```python
from build123d import *

# Parameters (mm, degrees)
SKETCH1_W           = 35.5
SKETCH1_H           = 37
SKETCH1_W_2         = 31.32
SKETCH1_H_2         = 15.62
BOSS_EXTRUDE1_DEPTH = 3
SKETCH2_W           = 35.5
SKETCH2_H           = 10
SKETCH2_R           = 1.65
BOSS_EXTRUDE2_DEPTH = 3


with BuildPart() as part:
    # Sketch1 → Boss-Extrude1 (new body)
    with BuildSketch(Plane.XY):
        with Locations((17.75, 18.5)):
            Rectangle(SKETCH1_W, SKETCH1_H)
        with BuildLine():
            Line((4.5, 35.95), (5.6, 35.95))
            ThreePointArc((5.6, 35.95), (6.7, 34.85), (5.6, 33.75))
            Line((5.6, 33.75), (4.5, 33.75))
            ThreePointArc((4.5, 33.75), (3.4, 34.85), (4.5, 35.95))
        make_face(mode=Mode.SUBTRACT)
        with BuildLine():
            Line((29.9, 35.95), (31, 35.95))
            ThreePointArc((31, 35.95), (32.1, 34.85), (31, 33.75))
            Line((31, 33.75), (29.9, 33.75))
            ThreePointArc((29.9, 33.75), (28.8, 34.85), (29.9, 35.95))
        make_face(mode=Mode.SUBTRACT)
        with BuildLine():
            Line((29.9, 8.25), (31, 8.25))
            ThreePointArc((31, 8.25), (32.1, 7.15), (31, 6.05))
            Line((31, 6.05), (29.9, 6.05))
            ThreePointArc((29.9, 6.05), (28.8, 7.15), (29.9, 8.25))
        make_face(mode=Mode.SUBTRACT)
        with BuildLine():
            Line((4.5, 8.25), (5.6, 8.25))
            ThreePointArc((5.6, 8.25), (6.7, 7.15), (5.6, 6.05))
            Line((5.6, 6.05), (4.5, 6.05))
            ThreePointArc((4.5, 6.05), (3.4, 7.15), (4.5, 8.25))
        make_face(mode=Mode.SUBTRACT)
        with Locations((17.75, 23.05)):
            Rectangle(SKETCH1_W_2, SKETCH1_H_2, mode=Mode.SUBTRACT)
    extrude(amount=BOSS_EXTRUDE1_DEPTH)

    # Sketch2 → Boss-Extrude2 (add)
    with BuildSketch(Plane.XZ):
        with Locations((17.75, 8)):
            Rectangle(SKETCH2_W, SKETCH2_H)
        with Locations(Location((3.75, 9, 0), (0, 0, 270))):
            Circle(SKETCH2_R, mode=Mode.SUBTRACT)
        with Locations(Location((31.75, 9, 0), (0, 0, 270))):
            Circle(SKETCH2_R, mode=Mode.SUBTRACT)
    extrude(amount=-BOSS_EXTRUDE2_DEPTH)


solid = part.part
```
Design review of the part built by this model. Coordinates are the model's own, in mm. A direction names the side the tool comes from. Give positions to 0.01 mm unless a question says otherwise; leave off trailing zeros. Order: outer loops, then holes, each group sorted by start corner. A loop starts at its lowest first (then second) coordinate and runs counter-clockwise, first axis right, second up. Notation, with made-up numbers: (11, 86.5) -> (25, 86.5) arc R23 ccw to (25, 97.5) -> close; hole circle Ø2 at (77, 12). An arc over 180 degrees is marked (long way). Write each question's results on one line, items separated by ' | '. Start each with the question number.
Q1. Add section C-C on y = 23. Give the boundary of the cut face in (x, z).
Q2. Add section D-D on y = 33. Give the boundary of the cut face in (x, z), and give its area (4 significant figures).
Q3. Mouldability with a two-part tool opening along X and no side actions: class faces 1 (the flat face through (30.4, 8.25, 1.5)), 2 (the flat face through (35.5, 15.7, 2.6)), 3 (the flat face through (18, 13, 3)) as +X half, -X half, draft (parallel to the pull), parting line (faces both ways), or undercut.
Q4. Add section A-A on x = 16. Give the boundary of the cut face in (y, z).
Q5. Wall thickness on L1, parallel to X at y = 0.75, z = 9; L2, parallel to Y at x = 20.5, z = 1.5; L3, parallel to X at y = 21.5, z = 1.5: over which ranges is each line inside the solid? List them lowest first. Write a range as from..to.
Q6. Machinability: for faces 4 (the cylindrical face through (3.4, 7.1, 1.5)), 5 (the flat face through (18, 3, 8)), 6 (the flat face through (18, 15, 0)), which of the approach directions +Z, -Z, +X, -X, +Y, -Y give a long, thin tool a straight path to every point of the face, cutting with its end or side? Answer none if there is none.
Q7. For pin 1 (3 mm diameter, centred on x = 3.75, z = 9, fed in from +Y); pin 2 (4.5 mm diameter, centred on x = 31.75, z = 9, fed in from +Y); pin 3 (1.5 mm diameter, centred on x = 8, y = 5, fed in from +Z), all flat-tipped, find the tip position at first contact; note any pin that passes through.
Q8. Add section B-B on z = 9. Give the boundary of the cut face in (x, y).
Found:
1) outline: (0, 0) -> (2.09, 0) -> (2.09, 3) -> (0, 3) -> close; (33.41, 0) -> (35.5, 0) -> (35.5, 3) -> (33.41, 3) -> close
2) outline: (0, 0) -> (35.5, 0) -> (35.5, 3) -> (0, 3) -> close | area: 106.5 mm2
3) face 1: undercut | face 2: +X half | face 3: draft
4) outline: (0, 0) -> (15.24, 0) -> (15.24, 3) -> (3, 3) -> (3, 13) -> (0, 13) -> close; (30.86, 0) -> (37, 0) -> (37, 3) -> (30.86, 3) -> close
5) L1: x = 0..2.1, 5.4..30.1, 33.4..35.5 | L2: y = 0..15.24, 30.86..37 | L3: x = 0..2.09, 33.41..35.5
6) face 4: +Z, -Z | face 5: +Z, +X, -X, +Y | face 6: -Z, +X, -X, +Y, -Y
7) pin 1: passes through | pin 2: stops at y = 3 | pin 3: stops at z = 3
8) outline: (0, 0) -> (2.1, 0) -> (2.1, 3) -> (0, 3) -> close; (5.4, 0) -> (30.1, 0) -> (30.1, 3) -> (5.4, 3) -> close; (33.4, 0) -> (35.5, 0) -> (35.5, 3) -> (33.4, 3) -> close
